Solid Edge part; units mm, degrees
sketch "Sketch1" plane through (0, 0, 0) normal (0, 0, 1) x (1, 0, 0)
  line L0 (-183.0017, -120) -> (-227.4217, -120)
  line L1 (-289.5811, -57.8353) -> (-227.4217, -120)
  line L2 (-289.5811, -57.8353) -> (-351.7458, 4.3295)
  line L3 (-351.7458, 129.7437) -> (-351.7458, 4.3295)
  line L4 (-351.7458, 129.7437) -> (-351.7458, 255.1579)
  line L5 (-289.4346, 317.4691) -> (-351.7458, 255.1579)
  line L6 (-289.4346, 317.4691) -> (-227.7006, 379.2031)
  line L7 (0, 379.2031) -> (-227.7006, 379.2031)
  line L8 (0, 379.2031) -> (0, 0)
  line L9 (0, 0) -> (-183.0017, 0)
  line L10 (-183.0017, 0) -> (-183.0017, -120)
  dimension "D1" = 183.0017
  dimension "D2" = 183.0017
  dimension "D3" = 289.4346
  dimension "D4" = 289.4346
  dimension "D5" = 351.7458
  dimension "D6" = 351.7458
  dimension "D7" = 289.5811
  dimension "D8" = 289.5811
extrude "Protrusion1" add sketch "Sketch1" along normal blind 5
mirror "Mirror1" about plane through (0, 0, 0) normal (1, 0, 0) of "Protrusion1"
sketch "Sketch2" plane through (0, 149.6016, 5) normal (0, 0, 1) x (1, 0, 0)
  circle A0 centre (150, 209.6016) radius 3.75
  circle A1 centre (-150, 209.6016) radius 3.75
extrude "Cutout1" cut sketch "Sketch2" against normal through all
sketch "Sketch3" plane through (0, 149.6016, 5) normal (0, 0, 1) x (1, 0, 0)
  circle A0 centre (-331.7458, 53.7221) radius 3.5
  circle A1 centre (-331.7458, -96.2779) radius 3.5
  dimension "D1" = 331.7458
  dimension "D2" = 331.7458
extrude "Cutout2" cut sketch "Sketch3" against normal through all
mirror "Mirror2" about plane through (0, 0, 0) normal (1, 0, 0) of "Cutout2"
sketch "Sketch4" plane through (0, 149.6016, 0) normal (0, 0, -1) x (-1, 0, 0)
  line L0 (-351.7458, -111.1142) -> (-193.1203, -269.6016)
  line L1 (-193.1203, -269.6016) -> (-227.4217, -269.6016)
  arc A0 (-351.7458, -145.2721) -> (-227.4217, -269.6016) centre (-220.2414, -138.0974) ccw
  line L2 (-351.7458, -111.1142) -> (-351.7458, -145.2721)
extrude "Protrusion2" add sketch "Sketch4" against normal up to vertex (5 mm away)
sketch "Sketch5" plane through (0, 149.6016, 0) normal (0, 0, -1) x (-1, 0, 0)
  line L0 (-227.7006, 229.6016) -> (-351.7458, 105.5563)
  arc A0 (-351.7458, 105.5563) -> (-227.7006, 229.6016) centre (-220.2564, 98.1121) cw
extrude "Protrusion3" add sketch "Sketch5" against normal up to vertex (5 mm away)
mirror "Mirror3" about plane through (0, 0, 0) normal (1, 0, 0) of "Protrusion3", "Protrusion2"
sketch "Sketch6" plane through (0, 0, 2.5) normal (0, -1, 0) x (1, 0, 0)
  line L0 (-183.0017, 2.5) -> (183.0017, 2.5)
  line L1 (183.0017, 2.5) -> (183.0017, -2.5)
  line L2 (183.0017, -2.5) -> (-183.0017, -2.5)
  line L3 (-183.0017, -2.5) -> (-183.0017, 2.5)
extrude "Extrusionsausprägung_11" add sketch "Sketch6" along normal blind 1.13
sketch "Sketch7" plane through (0, 129.6016, 5) normal (0, 0, 1) x (1, 0, 0)
  line L0 (-183.0017, -130.7316) -> (183.0017, -130.7316)
  line L1 (183.0017, -130.7316) -> (183.0017, -115.7316)
  line L2 (183.0017, -115.7316) -> (-183.0017, -115.7316)
  line L3 (-183.0017, -115.7316) -> (-183.0017, -130.7316)
  dimension "D1" = 183.0017
extrude "Cutout3" cut sketch "Sketch7" against normal through all
properties material "ABS-Plastik, mittelfest"
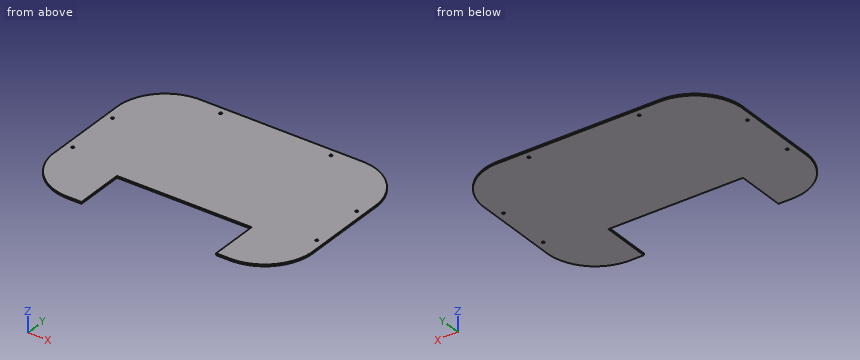
Input: part model. Units: mm. Frame: model coordinates. Coordinates: 2 decimals unless noted, no trailing zeros. Write each loop counter-clockwise with the first axis right and the second up, starting at its lowest first coordinate (ties: lowest second). Pieces come first, ordered by that corner, then holes. Notation, with made-up numbers: M -20,-32.5 L 11,-32.5 A21 ccw 11,-8.5 Z; hole C 30,60.5 d5. An arc over 180 degrees is marked long. Answer as a JSON object with one key per item and string values. Group by question number.
(1) Section C-C on x = -78. Output: boundary loops of the cut face in (y, z), plus the area to 3 significant figures.
(2) Section B-B on z = 4.25. Output: boundary loops of the cut face in (x, y), plus the area to 3 significant figures.
(3) Section D-D on x = -304. Output: boundary loops of the cut face in (y, z), plus the area to 3 significant figures.
(4) Contact query for flat-ended pins moving along their axis: P1, Ø1.5, axis at y = -46.5, z = 2.5, coming from the +X side; P2, Ø2.5, axis at x = 43, z = 3, coming from the -Y side; P3, Ø4.5, axis at x = 150, y = 359.2, coming from the +Z side. Output: stop coordinate, or through.
(5) Ray query, line 1 along X through (y, z) = (5, 3.6); line 2 along Y through (x, z) = (-150, 2.1); line 3 along X through (y, z) = (55, 4.8). Return the intervals inside material, ascending. Write a range as [from, to].
(6) Section A-A on y = -13. Output: boundary loops of the cut face in (x, z).
Result set:
{
 "1": {"outline": "M 13.87,0 L 379.2,0 L 379.2,5 L 13.87,5 Z", "area": "1,830 mm2"},
 "2": {"outline": "M -351.75,4.33 A131.7 ccw -227.42,-120 L -183,-120 L -183,13.87 L 183,13.87 L 183,-120 L 227.42,-120 A131.7 ccw 351.75,4.33 L 351.75,255.16 A131.7 ccw 227.7,379.2 L -227.7,379.2 A131.7 ccw -351.75,255.16 Z; hole C -331.75,53.32 d7; hole C -331.75,203.32 d7; hole C -150,359.2 d7.5; hole C 150,359.2 d7.5; hole C 331.75,53.32 d7; hole C 331.75,203.32 d7", "area": "287,000 mm2"},
 "3": {"outline": "M -90.13,0 L 349.36,0 L 349.36,5 L -90.13,5 Z", "area": "2,200 mm2"},
 "4": {"P1": "stops at x = 338.85", "P2": "stops at y = 13.87", "P3": "passes through"},
 "5": {"line 1": "x = [-351.75, -183], [183, 351.75]", "line 2": "y = [13.87, 355.45], [362.95, 379.2]", "line 3": "x = [-351.75, -334.82], [-328.67, 328.67], [334.82, 351.75]"},
 "6": {"outline": "M -349.64,0 L -183,0 L -183,5 L -349.64,5 Z; M 183,0 L 349.64,0 L 349.64,5 L 183,5 Z"}
}
